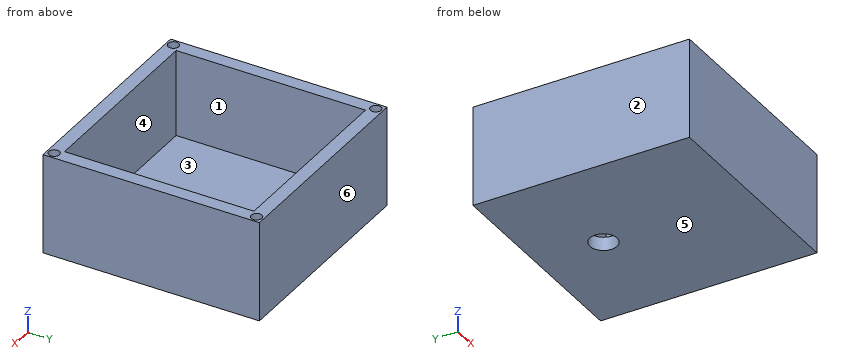
from build123d import *

# Parameters (mm, degrees)
SKETCH1_W           = 50.8
SKETCH1_H           = 50.8
BOSS_EXTRUDE1_DEPTH = 3.175
SKETCH3_W           = 50.8
SKETCH3_H           = 50.8
SKETCH3_W_2         = 44.4373
SKETCH3_H_2         = 44.45
BOSS_EXTRUDE2_DEPTH = 20.32
SKETCH4_R           = 3.175
CUT_EXTRUDE1_DEPTH  = 0.254
SKETCH6_R           = 1.2573
CUT_EXTRUDE2_DEPTH  = 9.525
SKETCH4_3_R         = 3.175
CUT_EXTRUDE3_DEPTH  = 75.66044736


with BuildPart() as part:
    # Sketch1 → Boss-Extrude1 (new body)
    with BuildSketch(Plane.XY):
        with Locations((25.4, 25.4)):
            Rectangle(SKETCH1_W, SKETCH1_H)
    extrude(amount=BOSS_EXTRUDE1_DEPTH)

    # Sketch3 → Boss-Extrude2 (add)
    with BuildSketch(Plane.XY.offset(3.175)):
        with Locations((25.4, 25.4)):
            Rectangle(SKETCH3_W, SKETCH3_H)
        with Locations((25.39365, 25.4)):
            Rectangle(SKETCH3_W_2, SKETCH3_H_2, mode=Mode.SUBTRACT)
    extrude(amount=BOSS_EXTRUDE2_DEPTH)

    # Sketch4 → Cut-Extrude1 (cut)
    with BuildSketch(Plane.XY.offset(3.175)):
        with Locations((25.39365, 17.145)):
            Circle(SKETCH4_R)
    extrude(amount=-CUT_EXTRUDE1_DEPTH, mode=Mode.SUBTRACT)

    # Sketch6 → Cut-Extrude2 (cut)
    with BuildSketch(Plane.XY.offset(23.495)):
        with Locations((1.651, 49.149)):
            Circle(SKETCH6_R)
        with Locations((49.149, 49.149)):
            Circle(SKETCH6_R)
        with Locations((49.149, 1.651)):
            Circle(SKETCH6_R)
        with Locations((1.651, 1.651)):
            Circle(SKETCH6_R)
    extrude(amount=-CUT_EXTRUDE2_DEPTH, mode=Mode.SUBTRACT)

    # Sketch4<3> → Cut-Extrude3 (cut, through all)
    with BuildSketch(Plane.XY.offset(3.175)):
        with Locations((25.39365, 35.1409)):
            Circle(SKETCH4_3_R)
    extrude(amount=-CUT_EXTRUDE3_DEPTH, mode=Mode.SUBTRACT)


solid = part.part
Part model, mm, in its own coordinate system. Face numbers are marked on the shaded views. A direction names the side the tool comes from. Give positions to 0.01 mm unless a question says otherwise; leave off trailing zeros. Loops run counter-clockwise (first coordinate to the right, second up) from the corner with the lowest first, then second, coordinate; pieces in that order, holes last. Notation, with made-up numbers: M -38,29 L 19,29 A25 cw 19,45 Z; hole C 41.25,-38.75 d2. An arc over 180 degrees is marked long. Put each result on its own line as item: value. Start each with the question number.
1) Pull direction Y, two halves, no side cores. Call the marked faces 3, 4, 5 and 6: +Y half, -Y half, draft (parallel to the pull), parting line (faces both ways), or undercut.
2) Flat gauge pins, fed straight in: pin 1 (3.5 mm diameter, centred on x = 49.149, y = 1.651, fed in from -Z); pin 2 (13.5 mm diameter, centred on x = 20, y = 32, fed in from +Z) (3 decimals); pin 3 (1.9 mm diameter, centred on x = 25.5, y = 18.5, fed in from +Z). Where does each tip first touch, or does it go through?
3) Saw through at A-A (z = 12). List the corners of the cut face in (x, y) (3 decimals).
4) Saw through at B-B (x = 23). List the corners of the cut face in (y, z) (3 decimals), then the cut area to 3 significant figures.
5) Saw through at D-D (x = 33). List the corners of the cut face in (y, z) (3 decimals), then the cut area to 3 significant figures.
6) 3-axis set-ups, long thin cutter, end or side, ignore diameter. For the marked faces 1 and 2: which of +Z, -Z, +X, -X, +Y, -Y reach the whole face in a straight line?
7) Probe probe 1 along Y at (x, z) = (43.5, 3.25) (3 decimals); probe 2 along X at (y, z) = (26.5, 16.25) (3 decimals); probe 3 along Z at (x, y) = (33.5, 46) (3 decimals). List the from-to ranges inside material, lowest first.
8) Saw through at C-C (y = 44). List the corners of the cut face in (x, z) (3 decimals), then the cut area to 3 significant figures.
Numbers:
1. face 3: undercut
1. face 4: undercut
1. face 5: draft
1. face 6: +Y half
2. pin 1: z = 0
2. pin 2: z = 3.175
2. pin 3: z = 2.92
3. outline: M 0,0 L 50.8,0 L 50.8,50.8 L 0,50.8 Z; hole M 3.175,3.175 L 47.612,3.175 L 47.612,47.625 L 3.175,47.625 Z
4. outline: M 0,0 L 33.055,0 L 33.055,3.175 L 19.231,3.175 L 19.231,2.921 L 15.059,2.921 L 15.059,3.175 L 3.175,3.175 L 3.175,23.495 L 0,23.495 Z; M 37.227,0 L 50.8,0 L 50.8,23.495 L 47.625,23.495 L 47.625,3.175 L 37.227,3.175 Z
4. area: 276 mm^2
5. outline: M 0,0 L 50.8,0 L 50.8,23.495 L 47.625,23.495 L 47.625,3.175 L 3.175,3.175 L 3.175,23.495 L 0,23.495 Z
5. area: 290 mm^2
6. face 1: +Z
6. face 2: +Z, -Z, -X, +Y, -Y
7. probe 1: 0 to 3.175, 47.625 to 50.8
7. probe 2: 0 to 3.175, 47.612 to 50.8
7. probe 3: 0 to 3.175
8. outline: M 0,0 L 50.8,0 L 50.8,23.495 L 47.612,23.495 L 47.612,3.175 L 3.175,3.175 L 3.175,23.495 L 0,23.495 Z
8. area: 291 mm^2
